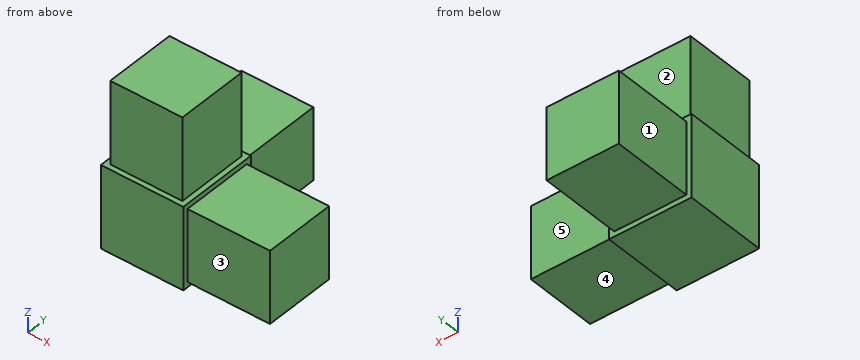
Autodesk Inventor part; units mm, degrees
ref_plane "YZ Plane" through (0, 0, 0) normal (1, 0, 0) x (0, 1, 0)
ref_plane "XZ Plane" through (0, 0, 0) normal (0, 1, 0) x (-1, 0, 0)
ref_plane "XY Plane" through (0, 0, 0) normal (0, 0, 1) x (1, 0, 0)
sketch "Sketch1" plane through (0, 0, 0) normal (0, 0, 1) x (1, 0, 0)
  line L0 (0, 0) -> (25.4, 0)
  line L1 (25.4, 0) -> (25.4, 25.4)
  line L2 (25.4, 25.4) -> (0, 25.4)
  line L3 (0, 25.4) -> (0, 0)
  line L4 (1.5875, 23.8125) -> (23.8125, 23.8125)
  line L5 (23.8125, 23.8125) -> (23.8125, 1.5875)
  line L6 (23.8125, 1.5875) -> (1.5875, 1.5875)
  line L7 (1.5875, 1.5875) -> (1.5875, 23.8125)
  dimension "d0" = 25.4
  dimension "d1" = 25.4
  dimension "d4" = 1.5875
extrude "Extrusion1" add sketch "Sketch1" against normal blind 25.4 contours L3 L2 L1 L0 | L4 L5 L6 L7
extrude "Extrusion2" add sketch "Sketch1" along normal blind 25.4 contours L4 L5 L6 L7
sketch "Sketch2" plane through (25.4, 0, 0) normal (1, 0, 0) x (0, 0, -1)
  line L0 (25.4, 0) -> (25.4, 25.4)
  line L1 (0, 25.4) -> (25.4, 25.4)
  line L2 (0, 0) -> (0, 25.4)
  line L3 (0, 0) -> (25.4, 0)
  line L4 (23.8125, 23.8125) -> (23.8125, 1.5875)
  line L5 (23.8125, 1.5875) -> (1.5875, 1.5875)
  line L6 (1.5875, 1.5875) -> (1.5875, 23.8125)
  line L7 (1.5875, 23.8125) -> (23.8125, 23.8125)
  dimension "d8" = 1.5875
sketch "Sketch3" plane through (0, 25.4, 0) normal (0, 1, 0) x (1, 0, 0)
  line L0 (25.4, 25.4) -> (0, 25.4)
  line L1 (0, 0) -> (0, 25.4)
  line L2 (25.4, 0) -> (0, 0)
  line L3 (25.4, 0) -> (25.4, 25.4)
  line L4 (1.5875, 23.8125) -> (23.8125, 23.8125)
  line L5 (23.8125, 23.8125) -> (23.8125, 1.5875)
  line L6 (23.8125, 1.5875) -> (1.5875, 1.5875)
  line L7 (1.5875, 1.5875) -> (1.5875, 23.8125)
  dimension "d9" = 1.5875
extrude "Extrusion3" add sketch "Sketch2" along normal blind 25.4 contours L4 L5 L6 L7
extrude "Extrusion4" add sketch "Sketch3" along normal blind 25.4 contours L4 L5 L6 L7
properties part number "3-way corner"
Work out the finished part from the listing and answer in its coordinate system (mm). Face numbers are marked on the shaded views. A direction names the side the tool comes from. Round coordinates to 2 decimals unless told otherwise and drop trailing zeros. Loops run counter-clockwise (first coordinate to the right, second up) from the corner with the lowest first, then second, coordinate; pieces in that order, holes last.
(1) The part is cut by section A-A, the plane z = -18. Give the vertices of the cut face in (x, y), and give its area (3 significant figures).
Computed values:
outline: (0, 0) - (25.4, 0) - (25.4, 1.59) - (50.8, 1.59) - (50.8, 23.81) - (25.4, 23.81) - (25.4, 25.4) - (23.81, 25.4) - (23.81, 50.8) - (1.59, 50.8) - (1.59, 25.4) - (0, 25.4) - close
area: 1,770 mm2
(2) The part is cut by section B-B, the plane y = 21. Give the vertices of the cut face in (x, z), and give its area (3 significant figures).
Computed values:
outline: (0, -25.4) - (25.4, -25.4) - (25.4, -23.81) - (50.8, -23.81) - (50.8, -1.59) - (25.4, -1.59) - (25.4, 0) - (23.81, 0) - (23.81, 25.4) - (1.59, 25.4) - (1.59, 0) - (0, 0) - close
area: 1,770 mm2
(3) For the marked faces 1, 2, 3, 4 and 5, determine the directions among +Z, -Z, +X, -X, +Y, -Y from which every point of the face is accessible in a straight line to the end or side of a thin tool.
Computed values:
face 1: +Z, -Z, -X, +Y
face 2: +Z, +X, -X, +Y
face 3: +Z, -Z, +X, -Y
face 4: -Z, +X, +Y, -Y
face 5: +Z, -Z, +X, +Y
(4) Find the intervals of material crossed by L1, parallel to Z at x = 33, y = 5.5; L2, parallel to Y at x = 34, z = -10.5, in increasing order.
Computed values:
L1: z = -23.81 to -1.59
L2: y = 1.59 to 23.81
(5) Each of these flat-tipped pins is pushed along its axis until it touches: P1, Ø5, axis at x = 34.5, y = 21, coming from the +Z side; P2, Ø11, axis at y = 39, z = -14.5, coming from the -X side; P3, Ø6.5, axis at x = 36.5, y = 15.5, coming from the -Z side. Where does it stop, or does it pass through?
Computed values:
P1: stops at z = -1.59
P2: stops at x = 1.59
P3: stops at z = -23.81
(6) The part is cut by section D-D, the plane z = 22.5. Give the vertices of the cut face in (x, y).
Computed values:
outline: (1.59, 1.59) - (23.81, 1.59) - (23.81, 23.81) - (1.59, 23.81) - close
(7) The part is cut by section C-C, the plane x = 28.5. Give the vertices of the cut face in (y, z), and give its area (3 significant figures).
Computed values:
outline: (1.59, -23.81) - (23.81, -23.81) - (23.81, -1.59) - (1.59, -1.59) - close
area: 494 mm2
